Input: dimensioned drawing with shaded views. Units: mm. Origin: part minimum x, y, z. A direction names the side the tool comes from. Round coordinates to 2 decimals unless told otherwise and drop trailing zeros. Order: outer loops, then holes, each group sorted by start corner. A loop starts at its lowest first (then second) coordinate and runs counter-clockwise, first axis right, second up. Notation, with made-up numbers: M 9,53.5 L 17,53.5 A23 cw 17,62.5 Z; hole C 43,49 d6. An arc over 180 degrees is marked long. One line per question, with ' | ' between items.
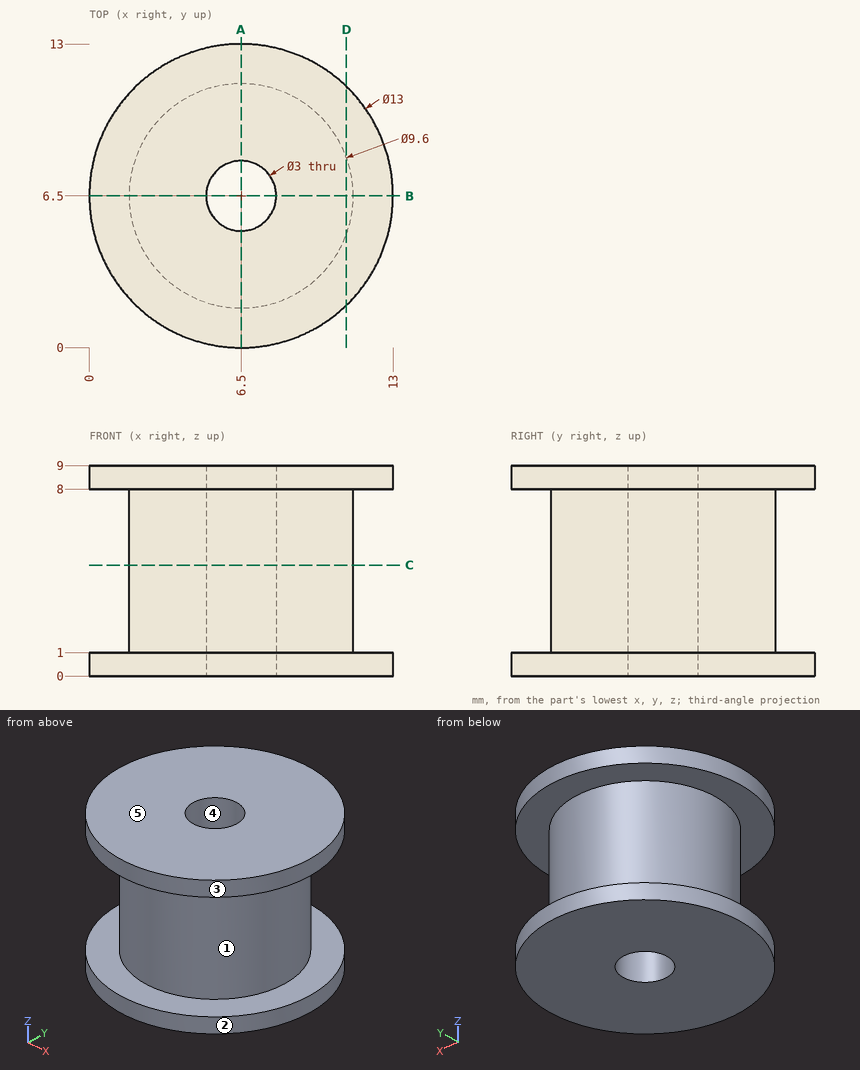
Item 1: Section query C-C, the plane z = 4.75. Return loops of the section in (x, y).
Report:
outline: C 6.5,6.5 d9.6; hole C 6.5,6.5 d3
Item 2: Mould query, pull axis X, two halves, no side actions, for the marked faces 3, 4 and 5. Classes: +X half, -X half, draft (parallel to the pull), parting line (faces both ways), or undercut.
Report:
face 3: parting line | face 4: undercut | face 5: draft
Item 3: Section query D-D, the plane x = 11. Return loops of the section in (y, z).
Report:
outline: M 1.81,0 L 11.19,0 L 11.19,1 L 8.17,1 L 8.17,8 L 11.19,8 L 11.19,9 L 1.81,9 L 1.81,8 L 4.83,8 L 4.83,1 L 1.81,1 Z
Item 4: Section query A-A, the plane x = 6.5. Return loops of the section in (y, z), plus the area to 3 significant figures.
Report:
outline: M 0,0 L 5,0 L 5,9 L 0,9 L 0,8 L 1.7,8 L 1.7,1 L 0,1 Z; M 8,0 L 13,0 L 13,1 L 11.3,1 L 11.3,8 L 13,8 L 13,9 L 8,9 Z | area: 66.2 mm²
Item 5: Line query: line 1 along Y through (x, z) = (6.5, 3.5); line 2 along Z through (x, y) = (8.25, 1); line 3 along X through (y, z) = (8.75, 6.25). Output: solid intervals per line, ascending. Write a range as from..to.
Report:
line 1: 1.7..5, 8..11.3 | line 2: 0..1, 8..9 | line 3: 2.26..10.74
Item 6: Access query for the marked faces 1 and 2. Directions: +Z, -Z, +X, -X, +Y, -Y. A direction counts if a zero-diameter tool reaches every point of the face in a straight line with its end or side. Return the directions, or none.
Report:
face 1: none | face 2: +Z, -Z
Item 7: First-contact query: pin 1 (1 mm diameter, centred on x = 6.5, z = 5, fed in from -Y); pin 2 (1 mm diameter, centred on y = 3, z = 4.5, fed in from +X); pin 3 (1.5 mm diameter, centred on y = 5.5, z = 5.5, fed in from +X). Flat tips, straight axial feed; report the tip coordinate or a pass-through.
Report:
pin 1: y = 1.7 | pin 2: x = 10.25 | pin 3: x = 11.29
